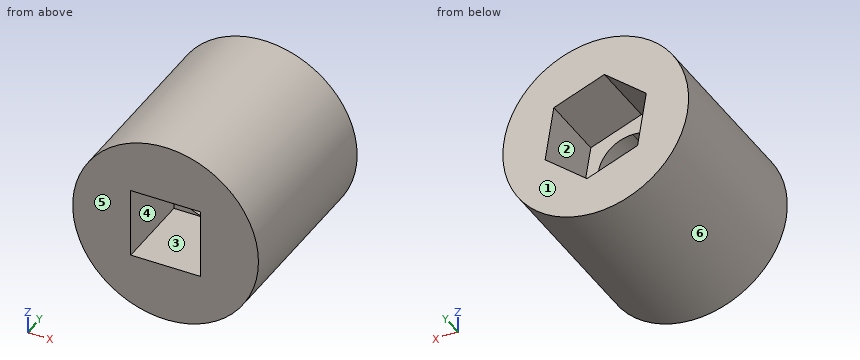
```python
from build123d import *

# Parameters (mm, degrees)
F0_R     = 12.7
F1_DEPTH = 25.4
F3_DEPTH = 25.401
F4_DEPTH = 11.0998
F6_DEPTH = 9.525


with BuildPart() as f1:
    # F0 (on Front) → F1 (new body)
    with BuildSketch(Plane.XZ):
        Circle(F0_R)
    extrude(amount=-F1_DEPTH)

    # F2 (on Front) → F3 (cut, through all)
    with BuildSketch(Plane.XZ):
        with BuildLine():
            ThreePointArc((-4.7625, 0), (-3.367596, -3.367596), (0, -4.7625))
            ThreePointArc((0, -4.7625), (3.367596, -3.367596), (4.7625, 0))
            ThreePointArc((4.7625, 0), (3.367596, 3.367596), (0, 4.7625))
            ThreePointArc((0, 4.7625), (-3.367596, 3.367596), (-4.7625, 0))
        make_face()
    extrude(amount=-F3_DEPTH, mode=Mode.SUBTRACT)

    # F2 (on Front) → F4 (cut)
    with BuildSketch(Plane.XZ):
        with BuildLine():
            Line((0, -4.7625), (4.7625, -4.7625))
            Line((4.7625, -4.7625), (4.7625, 0))
            ThreePointArc((4.7625, 0), (3.367596, -3.367596), (0, -4.7625))
        make_face()
        with BuildLine():
            Line((-4.7625, -4.7625), (0, -4.7625))
            ThreePointArc((0, -4.7625), (-3.367596, -3.367596), (-4.7625, 0))
            Line((-4.7625, 0), (-4.7625, -4.7625))
        make_face()
        with BuildLine():
            ThreePointArc((0, 4.7625), (3.367596, 3.367596), (4.7625, 0))
            Line((4.7625, 0), (4.7625, 4.7625))
            Line((4.7625, 4.7625), (0, 4.7625))
        make_face()
        with BuildLine():
            Line((-4.7625, 4.7625), (-4.7625, 0))
            ThreePointArc((-4.7625, 0), (-3.367596, 3.367596), (0, 4.7625))
            Line((0, 4.7625), (-4.7625, 4.7625))
        make_face()
    extrude(amount=-F4_DEPTH, mode=Mode.SUBTRACT)

    # F5 (on face) → F6 (cut)
    with BuildSketch(Plane(origin=(0, 25.4, 0), x_dir=(-1, 0, 0), z_dir=(0, 1, 0))):
        Polygon((-6.918703, -2.621455), (-1.189105, -7.3025), (5.729598, -4.681045), (6.918703, 2.621455), (1.189105, 7.3025), (-5.729598, 4.681045), align=None)
    extrude(amount=-F6_DEPTH, mode=Mode.SUBTRACT)


solid = f1.part
```
Read the model definition and answer for the solid it produces. Units are mm, in the model's axes. Face numbers are marked on the shaded views. A direction names the side the tool comes from. Coordinates: 2 decimals unless noted, no trailing zeros. Order: outer loops, then holes, each group sorted by start corner. A loop starts at its lowest first (then second) coordinate and runs counter-clockwise, first axis right, second up. Notation, with made-up numbers: (1.25, 88.5) - (11.25, 88.5) arc R19 ccw to (11.25, 113.5) - close; hole circle Ø7 at (0.25, 68.25). An arc over 180 degrees is marked (long way). Answer as a JSON object with one key per item and string values. Group by question number.
Item 1: Section C-C (y = 19.5) is taken. Give the vertices of the cut face in (x, z).
Item 2: Flat-ended cylindrical pins translate along their axes: P1, Ø12, axis at x = -1.5, y = 12.5, coming from the -Z side; P2, Ø4, axis at x = 2, z = 2, coming from the -Y side; P3, Ø3, axis at x = 2, y = 6, coming from the +Z side; P4, Ø1.5, axis at x = -9, y = 17.5, coming from the +Z side. Find the tip coordinate at first contact, or state that the pin passes through.
Item 3: Consider probe 1 along X at (y, z) = (14, -0.25); probe 2 along X at (y, z) = (18.5, -4.5); probe 3 along Z at (x, y) = (-1.75, 19.5). Determine where each line is inside the solid, lowest interval first. Write a range as from..to.
Item 4: The mould has two halves that part along Z. Classify the marked faces 4, 5 and 6: +Z half, -Z half, draft (parallel to the pull), parting line (faces both ways), or undercut.
Item 5: A tool of negligible diameter and unlimited length cuts with its end or side. For the marked faces 1, 2 and 3, from which of +Z, -Z, +X, -X, +Y, -Y can it reach the whole face along a straight path? Write none if from no direction.
Item 6: Section A-A (x = -3.5) is taken. Give the vertices of the cut face in (y, z) (1 decimal).
Item 7: Section B-B (y = 5.5) is taken. Give the vertices of the cut face in (x, z), plus the area to 3 significant figures.
Results are:
{
 "1": {"outline": "circle Ø25.4 at (0, 0); hole (-6.92, 2.62) - (-5.73, -4.68) - (1.19, -7.3) - (6.92, -2.62) - (5.73, 4.68) - (-1.19, 7.3) - close"},
 "2": {"P1": "stops at z = -12.7", "P2": "stops at y = 11.1", "P3": "stops at z = 12.69", "P4": "stops at z = 9.66"},
 "3": {"probe 1": "x = -12.7..-4.76, 4.76..12.7", "probe 2": "x = -11.88..-5.76, 4.62..11.88", "probe 3": "z = -12.58..-6.19, 6.84..12.58"},
 "4": {"face 4": "undercut", "face 5": "draft", "face 6": "parting line"},
 "5": {"face 1": "+Z, -Z, +X, -X, +Y", "face 2": "+Y", "face 3": "-Y"},
 "6": {"outline": "(0, -12.2) - (25.4, -12.2) - (25.4, -5.5) - (15.9, -5.5) - (15.9, -3.2) - (11.1, -3.2) - (11.1, -4.8) - (0, -4.8) - close; (0, 4.8) - (11.1, 4.8) - (11.1, 3.2) - (15.9, 3.2) - (15.9, 5.4) - (25.4, 5.4) - (25.4, 12.2) - (0, 12.2) - close"},
 "7": {"outline": "circle Ø25.4 at (0, 0); hole (-4.76, -4.76) - (4.76, -4.76) - (4.76, 4.76) - (-4.76, 4.76) - close", "area": "416 mm^2"}
}
